```python
from build123d import *

# Parameters (mm, degrees)
SKETCH1_W           = 22
SKETCH1_H           = 30
BOSS_EXTRUDE1_DEPTH = 10
SKETCH2_R           = 3
CUT_EXTRUDE1_DEPTH  = 44
SKETCH3_W           = 8.5
SKETCH3_H           = 30
BOSS_EXTRUDE2_DEPTH = 10
SKETCH4_W           = 1.5
SKETCH4_H           = 1
CUT_EXTRUDE2_DEPTH  = 8
SKETCH5_W           = 6.460308978
SKETCH5_H           = 15.152222924
BOSS_EXTRUDE3_DEPTH = 21
CHAMFER1_SIZE       = 1
FILLET1_R           = 5


with BuildPart() as part:
    # Sketch1 → Boss-Extrude1 (new body)
    with BuildSketch(Plane.XY):
        Rectangle(SKETCH1_W, SKETCH1_H)
    extrude(amount=BOSS_EXTRUDE1_DEPTH)

    # Sketch2 → Cut-Extrude1 (cut)
    with BuildSketch(Plane(origin=(0, 15, 0), x_dir=(1, 0, 0), z_dir=(0, 1, 0))):
        with Locations(Location((-6, -4.824366767, 0), (0, 0, 270))):
            Circle(SKETCH2_R)
        with Locations(Location((6, -4.824366767, 0), (0, 0, 270))):
            Circle(SKETCH2_R)
    extrude(amount=-CUT_EXTRUDE1_DEPTH, mode=Mode.SUBTRACT)

    # Sketch3 → Boss-Extrude2 (add)
    with BuildSketch(Plane.XY.offset(10)):
        with Locations((-6.75, 0)):
            Rectangle(SKETCH3_W, SKETCH3_H)
    extrude(amount=BOSS_EXTRUDE2_DEPTH)

    # Sketch4 → Cut-Extrude2 (cut)
    with BuildSketch(Plane.XY.offset(18)):
        Polygon((-10.5, 14), (-10.5, 15), (-11, 15), (-11, -15), (-10.5, -15), (-10.5, -14), (-10.5, -13), (-10.5, -12), (-10.5, -11), (-10.5, -10), (-10.5, -9), (-10.5, -8), (-10.5, -7), (-10.5, -6), (-10.5, -5), (-10.5, -4), (-10.5, -3), (-10.5, -2), (-10.5, -1), (-10.5, 0), (-10.5, 1), (-10.5, 2), (-10.5, 3), (-10.5, 4), (-10.5, 5), (-10.5, 6), (-10.5, 7), (-10.5, 8), (-10.5, 9), (-10.5, 10), (-10.5, 11), (-10.5, 12), (-10.5, 13), align=None)
        with Locations((-9.75, 13.5)):
            Rectangle(SKETCH4_W, SKETCH4_H)
        with Locations((-9.75, 11.5)):
            Rectangle(SKETCH4_W, SKETCH4_H)
        with Locations((-9.75, 9.5)):
            Rectangle(SKETCH4_W, SKETCH4_H)
        with Locations((-9.75, 7.5)):
            Rectangle(SKETCH4_W, SKETCH4_H)
        with Locations((-9.75, 5.5)):
            Rectangle(SKETCH4_W, SKETCH4_H)
        with Locations((-9.75, 3.5)):
            Rectangle(SKETCH4_W, SKETCH4_H)
        with Locations((-9.75, 1.5)):
            Rectangle(SKETCH4_W, SKETCH4_H)
        with Locations((-9.75, -0.5)):
            Rectangle(SKETCH4_W, SKETCH4_H)
        with Locations((-9.75, -2.5)):
            Rectangle(SKETCH4_W, SKETCH4_H)
        with Locations((-9.75, -4.5)):
            Rectangle(SKETCH4_W, SKETCH4_H)
        with Locations((-9.75, -6.5)):
            Rectangle(SKETCH4_W, SKETCH4_H)
        with Locations((-9.75, -8.5)):
            Rectangle(SKETCH4_W, SKETCH4_H)
        with Locations((-9.75, -10.5)):
            Rectangle(SKETCH4_W, SKETCH4_H)
        with Locations((-9.75, -12.5)):
            Rectangle(SKETCH4_W, SKETCH4_H)
        with Locations((-9.75, -14.5)):
            Rectangle(SKETCH4_W, SKETCH4_H)
    extrude(amount=-CUT_EXTRUDE2_DEPTH, mode=Mode.SUBTRACT)

    # Sketch5 → Boss-Extrude3 (add)
    with BuildSketch(Plane(origin=(0, 0, 0), x_dir=(-1, 0, 0), z_dir=(0, 0, -1))):
        Rectangle(SKETCH5_W, SKETCH5_H)
    extrude(amount=BOSS_EXTRUDE3_DEPTH)

    # Chamfer1
    chamfer1_edges = [part.edges().sort_by_distance(p)[0] for p in [
        (-6, -15, 1.824366767),
        (-6, 15, 1.824366767),
        (6, -15, 1.824366767),
        (6, 15, 1.824366767),
    ]]
    chamfer(chamfer1_edges, length=CHAMFER1_SIZE)

    # Fillet1
    fillet1_edges = [part.edges().sort_by_distance(p)[0] for p in [
        (-2.5, 0, 20),
    ]]
    fillet(fillet1_edges, radius=FILLET1_R)


solid = part.part
```
Source: CAD feature listing. Evaluate the final solid. Frame: model axes, mm. A direction names the side the tool comes from. Coordinates: 2 decimals unless noted, no trailing zeros. Loops run counter-clockwise (first coordinate to the right, second up) from the corner with the lowest first, then second, coordinate; pieces in that order, holes last. Notation, with made-up numbers: M 56.5,-1 L 69.5,-1 A24 cw 69.5,16 Z; hole C 4.5,-32.5 d2. An arc over 180 degrees is marked long. Put each result on its own line as item: value. Start each with the question number.
1) Cut plane D-D on z = -3.5. Return the cut outline in (x, y).
2) Reachability of faces 1 (the face through (-10.5, 14.5, 14.1)), 2 (the face through (-9, 9.5, 14.1)), 3 (the face through (-9, 0, 20)) from +Z, -Z, +X, -X, +Y, -Y: full face, straight path, thin tool, end or side. Return the list, or none.
3) Cut plane C-C on x = 1.5. Return the cut outline in (y, z), then the cut area to 3 significant figures.
4) Cut plane A-A on x = 6. Return the cut outline in (y, z).
5) Cut plane B-B on y = -5.5. Return the cut outline in (x, z).
6) Pull-direction query (Z, two-part tool) for faces 4 (the face through (-3.93, 0.21, 18.5)), 5 (the face through (-9, 7.5, 14.1)), 6 (the face through (0, 7.576, -10)); classes: pulls with the +Z half, pulls with the -Z half, needs draft (parallel to the pull), parting line crosses it, or undercut.
7) Ray query, L1, parallel to X at y = 7.25, z = 7; L2, parallel to X at y = 5.25, z = 3; L3, parallel to X at y = 1, z = -9. Return the intervals inside material, ascending. Write a range as from..to.
8) Contact query for flat-ended pins moving along their axis: pin 1 Ø2 at (x, y) = (7.5, -10) entering from -Z; pin 2 Ø0.5 at (y, z) = (-12.5, 13) entering from -X; pin 3 Ø0.8 at (y, z) = (-1.5, 14.5) entering from -X; pin 4 Ø8 at (x, z) = (0, 13) entering from +Y. Output: stop coordinate, or through.
The answers:
1. outline: M -3.23,-7.58 L 3.23,-7.58 L 3.23,7.58 L -3.23,7.58 Z
2. face 1: -X, +Y, -Y
2. face 2: -X
2. face 3: +Z, +X, -X, +Y, -Y
3. outline: M -15,0 L -7.58,0 L -7.58,-21 L 7.58,-21 L 7.58,0 L 15,0 L 15,10 L -15,10 Z
3. area: 618 mm²
4. outline: M -15,0 L 15,0 L 15,0.82 L 14,1.82 L -14,1.82 L -15,0.82 Z; M -15,8.82 L -14,7.82 L 14,7.82 L 15,8.82 L 15,10 L -15,10 Z
5. outline: M -11,0 L -3.23,0 L -3.23,-21 L 3.23,-21 L 3.23,0 L 11,0 L 11,10 L -2.5,10 L -2.5,15 A5 ccw -7.5,20 L -11,20 L -11,18 L -10.5,18 L -10.5,10 L -11,10 Z; hole C -6,4.82 d6; hole C 6,4.82 d6
6. face 4: pulls with the +Z half
6. face 5: undercut
6. face 6: needs draft
7. L1: x = -11..-8.07, -3.93..3.93, 8.07..11
7. L2: x = -11..-8.38, -3.62..3.62, 8.38..11
7. L3: x = -3.23..3.23
8. pin 1: stops at z = 0
8. pin 2: stops at x = -9
8. pin 3: stops at x = -10.5
8. pin 4: stops at y = 15
